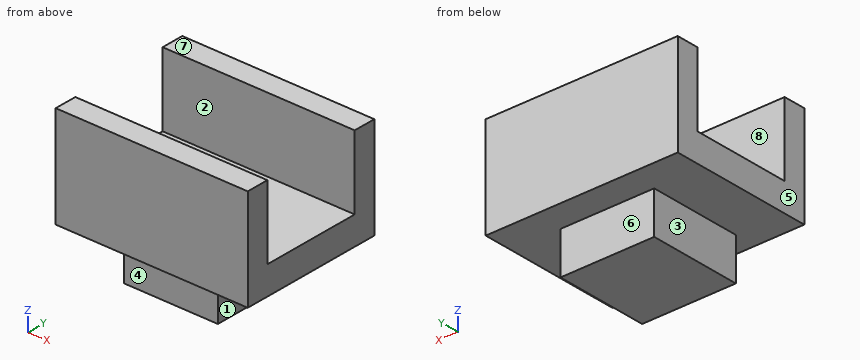
Autodesk Inventor part; units mm, degrees
ref_plane "YZ Plane" through (0, 0, 0) normal (1, 0, 0) x (0, 1, 0)
ref_plane "XZ Plane" through (0, 0, 0) normal (0, 1, 0) x (-1, 0, 0)
ref_plane "XY Plane" through (0, 0, 0) normal (0, 0, 1) x (1, 0, 0)
sketch "스케치1" plane through (0, 0, 0) normal (0, 0, 1) x (1, 0, 0)
  line L0 (-10.25, -7.75) -> (10.25, -7.75)
  line L1 (10.25, -7.75) -> (10.25, 7.75)
  line L2 (10.25, 7.75) -> (-10.25, 7.75)
  line L3 (-10.25, 7.75) -> (-10.25, -7.75)
  line L4 (-10.25, -7.75) -> (10.25, 7.75) construction
  line L5 (10.25, -7.75) -> (-10.25, 7.75) construction
  point P0 (0, 0)
  dimension "d0" = 20.5
  dimension "d1" = 15.5
extrude "돌출1" add sketch "스케치1" along normal blind 3
sketch "스케치2" plane through (0, 0, 3) normal (0, 0, 1) x (1, 0, 0)
  line L0 (10.25, 7.75) -> (-10.25, 7.75)
  line L1 (-10.25, 7.75) -> (10.25, 7.75)
  line L2 (10.25, 7.75) -> (10.25, 5.35)
  line L3 (10.25, 5.35) -> (-10.25, 5.35)
  line L4 (-10.25, 5.35) -> (-10.25, 7.75)
  line L5 (0, 0) -> (4.2226, 0)
  line L6 (10.25, -7.75) -> (-10.25, -7.75)
  line L7 (-10.25, -7.75) -> (10.25, -7.75)
  line L8 (10.25, -7.75) -> (10.25, -5.35)
  line L9 (10.25, -5.35) -> (-10.25, -5.35)
  line L10 (-10.25, -5.35) -> (-10.25, -7.75)
  dimension "d4" = 2.4
extrude "돌출2" add sketch "스케치2" along normal blind 7.8
sketch "스케치3" plane through (0, 0, 0) normal (0, 0, -1) x (-1, 0, 0)
  line L0 (-5, -5.3868) -> (5, -5.3868)
  line L1 (5, -5.3868) -> (5, 4.6132)
  line L2 (5, 4.6132) -> (-5, 4.6132)
  line L3 (-5, 4.6132) -> (-5, -5.3868)
  line L4 (-5, -5.3868) -> (5, 4.6132) construction
  line L5 (5, -5.3868) -> (-5, 4.6132) construction
  point P0 (0, 0)
  point P1 (0, -0.3868)
  dimension "d7" = 10
  dimension "d8" = 10
extrude "돌출3" add sketch "스케치3" along normal blind 4.5
properties part number "스텝모터 드라이버"
Design review of the part built by this model. Coordinates are the model's own, in mm. Face numbers are marked on the shaded views. A direction names the side the tool comes from. Give positions to 0.01 mm unless a question says otherwise; leave off trailing zeros. Order: outer loops, then holes, each group sorted by start corner. A loop starts at its lowest first (then second) coordinate and runs counter-clockwise, first axis right, second up. Notation, with made-up numbers: (-0.5, -28) - (40.5, -28) arc R3 ccw to (40.5, -24) - close; hole circle Ø10 at (77.25, -2). An arc over 180 degrees is marked (long way). Use CSV: the item, a comma, the result in double quotes. Start each with the question number.
Q1. Take a section at C-C (x = 4.5). State the section outline as (y, z) points.
Q2. Take a section at B-B (y = -1.75). State the section outline as (x, z) points.
Q3. For P1, Ø5, axis at x = -2, z = -1.5, coming from the +Y side; P2, Ø5.5, axis at x = 5, y = 1, coming from the +Z side; P3, Ø1.3, axis at y = 0.5, z = -2.5, coming from the +X side; P4, Ø1.5, axis at y = -2.5, z = -2.5, coming from the -X side, all flat-tipped, find the tip position at first contact; note any pin that passes through.
Q4. Machinability: for the marked faces 1, 2, 3, 4 and 5, which of the approach directions +Z, -Z, +X, -X, +Y, -Y give a long, thin tool a straight path to every point of the face, cutting with its end or side? Answer none if there is none.
Q5. Take a section at D-D (z = -0.25). State the section outline as (x, y) points, and give its area (3 significant figures).
Q6. For line 1 (Y direction, x = -5, z = 7); line 2 (Z direction, x = -4.75, y = -2.75); line 3 (X direction, y = -1.75, z = -1), list the stretches that pass through material, from the lowest coordinate up.
Q7. Draft analysis for pull direction Y (two halves, no side actions). For the marked faces 6, 7 and 8, state which applies: pulls with the +Y half, pulls with the -Y half, needs draft (parallel to the pull), parting line crosses it, or undercut.
Q8. Take a section at A-A (z = 6.5). State the section outline as (x, y) points, and give its area (3 significant figures).
Calculated:
1,outline,"(-7.75, 0) - (-5.39, 0) - (-5.39, -4.5) - (4.61, -4.5) - (4.61, 0) - (7.75, 0) - (7.75, 10.8) - (5.35, 10.8) - (5.35, 3) - (-5.35, 3) - (-5.35, 10.8) - (-7.75, 10.8) - close"
2,outline,"(-10.25, 0) - (-5, 0) - (-5, -4.5) - (5, -4.5) - (5, 0) - (10.25, 0) - (10.25, 3) - (-10.25, 3) - close"
3,P1,"stops at y = 7.75"
3,P2,"stops at z = 3"
3,P3,"stops at x = 5"
3,P4,"stops at x = -5"
4,face 1,"-Z, +X, +Y, -Y"
4,face 2,"+Z, +X, -X"
4,face 3,"-Z, -X, +Y, -Y"
4,face 4,"-Z, +X, -X, -Y"
4,face 5,"+Z, -Z, -X, +Y, -Y"
5,outline,"(-5, -5.39) - (5, -5.39) - (5, 4.61) - (-5, 4.61) - close"
5,area,"100 mm²"
6,line 1,"y = -7.75 to -5.35, 5.35 to 7.75"
6,line 2,"z = -4.5 to 3"
6,line 3,"x = -5 to 5"
7,face 6,"pulls with the +Y half"
7,face 7,"needs draft"
7,face 8,"undercut"
8,outline,"(-10.25, -7.75) - (10.25, -7.75) - (10.25, -5.35) - (-10.25, -5.35) - close; (-10.25, 5.35) - (10.25, 5.35) - (10.25, 7.75) - (-10.25, 7.75) - close"
8,area,"98.4 mm²"
